from build123d import *

# Parameters (mm, degrees)
EXTRUDE_THIN1_DEPTH = 170


with BuildPart() as part:
    # Sketch1 → Extrude-Thin1 (new body)
    with BuildSketch(Plane.XY):
        with BuildLine():
            Line((-100, 7.75), (0, 7.75))
            ThreePointArc((0, 7.75), (7.75, 0), (0, -7.75))
            Line((0, -7.75), (0, -19.75))
            ThreePointArc((0, -19.75), (19.75, 0), (0, 19.75))
            Line((0, 19.75), (-100, 19.75))
            Line((-100, 19.75), (-100, 7.75))
        make_face()
    extrude(amount=EXTRUDE_THIN1_DEPTH)


solid = part.part
Check sheet for the modelled part. Datum: model origin and axes. Units: mm. A direction names the side the tool comes from. Coordinates: 2 decimals unless noted, no trailing zeros. Write each loop counter-clockwise with the first axis right and the second up, starting at its lowest first coordinate (ties: lowest second). Pieces come first, ordered by that corner, then holes.
Item 1: Scan lines: probe 1 along Y at (x, z) = (-76, 121.5); probe 2 along Y at (x, z) = (1, 138.5); probe 3 along X at (y, z) = (-3.5, 23.5). Record each from-to range of solid material in increasing order.
Numbers:
probe 1: y = 7.75 to 19.75
probe 2: y = -19.72 to -7.69, 7.69 to 19.72
probe 3: x = 6.91 to 19.44
Item 2: Cross-section at A-A on x = 6. Record the boundary of the cut face in (y, z).
Numbers:
outline: (-18.82, 0) - (-4.91, 0) - (-4.91, 170) - (-18.82, 170) - close; (4.91, 0) - (18.82, 0) - (18.82, 170) - (4.91, 170) - close
Item 3: Mould release check, pull along Y, two halves, no side actions. Record for faces 1 (the face through (7.75, 0.17, 83.81)), 2 (the face through (-51, 7.75, 84)), 3 (the face through (-28, 9, 0)), 4 (the face through (-49, 19.75, 84)): released by +Y, released by -Y, zero draft, split by the parting line, or undercut.
Numbers:
face 1: undercut
face 2: released by -Y
face 3: zero draft
face 4: released by +Y
Item 4: Cross-section at B-B on z = 153. Record the boundary of the cut face in (x, y).
Numbers:
outline: (-100, 7.75) - (0, 7.75) arc R7.75 cw to (0, -7.75) - (0, -19.75) arc R19.75 ccw to (0, 19.75) - (-100, 19.75) - close
Item 5: Access from +Z, -Z, +X, -X, +Y, -Y to the whole of each face (thin tool, end or side, straight path). Record for faces 5 (the face through (19.745, -0.434, 83.81)), 6 (the face through (0, -14, 84)).
Numbers:
face 5: +Z, -Z, +X
face 6: +Z, -Z, -X, -Y
Item 6: Cross-section at C-C on x = -73.5. Record the boundary of the cut face in (y, z), then the cut area to 3 significant figures.
Numbers:
outline: (7.75, 0) - (19.75, 0) - (19.75, 170) - (7.75, 170) - close
area: 2,040 mm2
Item 7: Depth check by flat-ended pin: pin 1 Ø10 at (x, y) = (-24.5, 14) entering from -Z; pin 2 Ø13 at (y, z) = (-14, 54.5) entering from -X; pin 3 Ø4 at (x, z) = (-42.5, 78.5) entering from -Y. Enter the tip coordinate at first touch or a pass-through.
Numbers:
pin 1: stops at z = 0
pin 2: stops at x = 0
pin 3: stops at y = 7.75
